from build123d import *
from build123d.topology import SkipClean

# Parameters (mm, degrees)
SKETCH_1_R               = 4.5
SKETCH_1_R_2             = 3
EXTRUDE_1_DEPTH          = 9
CUT_EXTRUDE_3_DEPTH      = 12.022703843
CUT_EXTRUDE_3_DEPTH_BACK = 12.022703843
SKETCH_2_R               = 1
EXTRUDE_2_DEPTH          = 1


with BuildPart() as part:
    # ｽｹｯﾁ1 → ﾎﾞｽ - 押し出し1 (new body)
    with BuildSketch(Plane(origin=(0, 0, 0), x_dir=(1, 0, 0), z_dir=(0, 1, 0))):
        with Locations(Location((0, 0, 0), (0, 0, 270))):
            Circle(SKETCH_1_R)
        with Locations(Location((0, 0, 0), (0, 0, 270))):
            Circle(SKETCH_1_R_2, mode=Mode.SUBTRACT)
    extrude(amount=EXTRUDE_1_DEPTH)

    # ｽｹｯﾁ2 → ｶｯﾄ - 押し出し3 (cut, two sides: drawn at the far end of the back side and taken through both)
    with BuildSketch(Plane(origin=(0, 0, 0), x_dir=(0, 0, -1), z_dir=(1, 0, 0)).offset(-CUT_EXTRUDE_3_DEPTH_BACK)):
        with Locations((0, 9)):
            Circle(SKETCH_2_R)
    extrude(amount=CUT_EXTRUDE_3_DEPTH + CUT_EXTRUDE_3_DEPTH_BACK, mode=Mode.SUBTRACT)

    # ｽｹｯﾁ3 → ﾎﾞｽ - 押し出し2 (add)
    with SkipClean():  # the faces are left unmerged after this step: merging them gives an invalid solid
        with BuildSketch(Plane(origin=(0, 9, 0), x_dir=(1, 0, 0), z_dir=(0, 1, 0))):
            with BuildLine():
                Line((-2.828427125, -1), (-4.387482194, -1))
                ThreePointArc((-4.387482194, -1), (0, -4.5), (4.387482194, -1))
                Line((4.387482194, -1), (2.828427125, -1))
                ThreePointArc((2.828427125, -1), (0, -3), (-2.828427125, -1))
            make_face()
            with BuildLine():
                Line((2.828427125, 1), (4.387482194, 1))
                ThreePointArc((4.387482194, 1), (0, 4.5), (-4.387482194, 1))
                Line((-4.387482194, 1), (-2.828427125, 1))
                ThreePointArc((-2.828427125, 1), (0, 3), (2.828427125, 1))
            make_face()
        extrude(amount=EXTRUDE_2_DEPTH)


solid = part.part
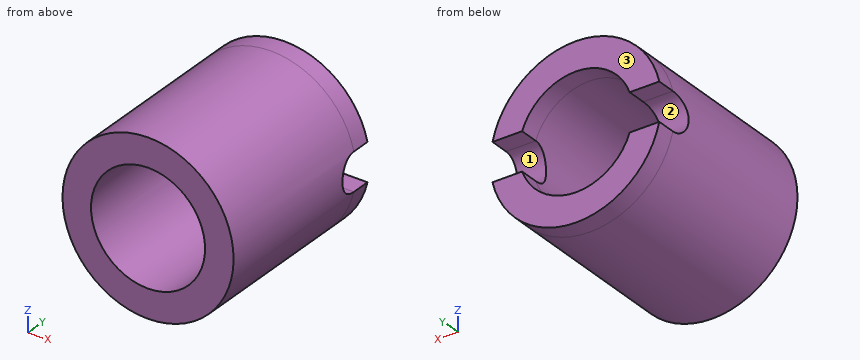
Model file for the job. Use its own axes, mm. Face numbers are marked on the shaded views. Give positions to 0.01 mm unless a question says otherwise; leave off trailing zeros. Loops run counter-clockwise (first coordinate to the right, second up) from the corner with the lowest first, then second, coordinate; pieces in that order, holes last. Notation, with made-up numbers: (-25.5, -19) - (-8.5, -19) arc R23 cw to (-8.5, 20) - close; hole circle Ø10 at (87, -12). An arc over 180 degrees is marked (long way). Use one line per item in the form item = value.
(1) Drop flat-ended pins along their axis: P1, Ø2, axis at y = 2.5, z = -3.5, coming from the +X side; P2, Ø1, axis at x = 3.5, y = 1.5, coming from the +Z side; P3, Ø0.8, axis at x = -4, y = 9.5, coming from the +Z side. Give the stop position or say it passes through.
Determined:
P1 = 3.74
P2 = 3.35
P3 = 2.7
(2) Drill centre lines: L1, parallel to Z at x = 0, y = 5; L2, parallel to Z at x = 2, y = 4.25. Where is each one in solid material? Low to high.
Determined:
L1 = -4.5 to -3, 3 to 4.5
L2 = -4.03 to -2.24, 2.24 to 4.03
(3) Cut at C-C (x = 0.5). Give the cut face in (y, z).
Determined:
outline = (0, -4.47) - (10, -4.47) - (10, -2.96) - (0, -2.96) - close; (0, 2.96) - (10, 2.96) - (10, 4.47) - (0, 4.47) - close
(4) Cut at D-D (y = 4). Give the cut face in (x, z), then the cut area to 3 significant figures.
Determined:
outline = circle Ø9 at (0, 0); hole circle Ø6 at (0, 0)
area = 35.3 mm^2
(5) Cut at B-B (z = -3.5). Give the cut face in (x, y).
Determined:
outline = (-2.83, 0) - (2.83, 0) - (2.83, 10) - (-2.83, 10) - close
(6) Cut at A-A (z = 0). Give the cut face in (x, y), then the cut area to 3 significant figures.
Determined:
outline = (-4.5, 0) - (-3, 0) - (-3, 8) - (-4.5, 8) - close; (3, 0) - (4.5, 0) - (4.5, 8) - (3, 8) - close
area = 24.0 mm^2
(7) Pull direction Z, two halves, no side cores. Call the marked faces 1, 2 and 3: pulls with the +Z half, pulls with the -Z half, needs draft (parallel to the pull), parting line crosses it, or undercut.
Determined:
face_1 = undercut
face_2 = undercut
face_3 = needs draft
